Autodesk Inventor part; units mm, degrees
ref_plane "YZ Plane" through (0, 0, 0) normal (1, 0, 0) x (0, 1, 0)
ref_plane "XZ Plane" through (0, 0, 0) normal (0, 1, 0) x (-1, 0, 0)
ref_plane "XY Plane" through (0, 0, 0) normal (0, 0, 1) x (1, 0, 0)
sketch "Sketch1" plane through (0, 0, 0) normal (0, 1, 0) x (-1, 0, 0)
  line L0 (0, 0) -> (25, 0)
  line L1 (0, -25) -> (0, 0)
  line L2 (25, 0) -> (50, 0)
  circle A0 centre (37.5, -12.5) radius 1.5
  circle A1 centre (12.5, -12.5) radius 1.5
  circle A2 centre (12.5, -37.5) radius 1.5
  line L3 (0, 0) -> (0, -25.5)
  line L4 (50, 0) -> (51, 0)
  line L5 (46.5711, -25.5) -> (39.5, -25.5)
  line L6 (25.5, -39.5) -> (25.5, -46.5711)
  line L7 (0, 0) -> (0, -65)
  line L8 (0, 0) -> (65, 0)
  line L9 (65, 0) -> (0, -65)
  line L10 (25.5, 0) -> (25.5, 5)
  line L11 (25.5, 5) -> (33.9376, 5)
  line L12 (0, -25.5) -> (-5, -25.5)
  line L13 (-5, -25.5) -> (-5, -33.9376)
  line L14 (32.5, -32.5) -> (36.0355, -36.0355)
  line L15 (36.0355, -36.0355) -> (25.5, -46.5711)
  line L16 (36.0355, -36.0355) -> (46.5711, -25.5)
  line L17 (28.9376, 0) -> (33.9376, 5)
  line L18 (-5, -33.9376) -> (0, -28.9376)
  line L19 (12.5, -12.5) -> (12.5, -37.5)
  line L20 (12.5, -12.5) -> (37.5, -12.5)
  line L21 (33.9376, 5) -> (38.9376, 0)
  line L22 (25.5, 5) -> (20.5, 0)
  line L23 (-5, -25.5) -> (0, -20.5)
  line L24 (-5, -33.9376) -> (0, -38.9376)
  line L25 (25.5, -46.5711) -> (18.4289, -46.5711)
  line L26 (46.5711, -25.5) -> (46.5711, -18.4289)
  line L27 (46.5711, -18.4289) -> (39.5, -25.5)
  line L28 (25.5, -39.5) -> (18.4289, -46.5711)
  line L29 (0, -20.5) -> (0, -25.5)
  line L30 (25.5, 0) -> (20.5, 0)
  line L31 (0, -28.9376) -> (0, -38.9376)
  line L32 (0, -20.5) -> (0, -25.5)
  line L33 (0, -25.5) -> (0, -28.9376)
  line L34 (0, -28.9376) -> (0, -38.9376)
  line L35 (-5, -33.9376) -> (0, -38.9376)
  line L36 (0, -38.9376) -> (0, -28.9376)
  line L37 (0, -28.9376) -> (-5, -33.9376)
  dimension "d36" = 25
  dimension "d38" = 25
  dimension "d42" = 3
  dimension "d43" = 3
  dimension "d44" = 3
  dimension "d45" = 25.5
  dimension "d47" = 1
  dimension "d51" = 65
  dimension "d52" = 65
  dimension "d54" = 5
  dimension "d55" = 5
  dimension "d56" = 5
extrude "Extrusion5" add sketch "Sketch1" along normal blind 2.5 contours L0 L2 L4 L8 L9 L7 L3 L1 | L22 L10 L2 L0 | L1 L3 L12 L23 | L21 L2 L17 | L18 L7 L24 | L9 L6 L25 | L26 L5 L9
extrude "Extrusion6" add sketch "Sketch1" along normal blind 8 contours L11 L17 L2 L10 | L12 L7 L18 L13 | L9 L14 L15 L6 | L9 L5 L16 L14
properties part number "stencil"
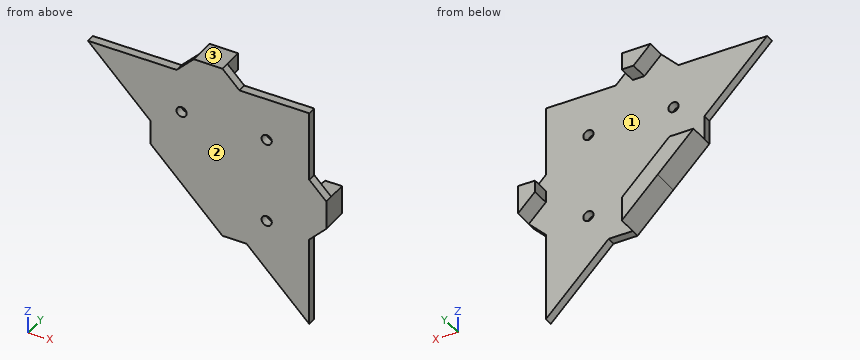
Design review of the part built by this model. Coordinates are the model's own, in mm. Face numbers are marked on the shaded views. Coordinates: 2 decimals unless noted, no trailing zeros. Order: outer loops, then holes, each group sorted by start corner. A loop starts at its lowest first (then second) coordinate and runs counter-clockwise, first axis right, second up. Notation, with made-up numbers: (32, -23.5) -> (52, -23.5) arc R5 cw to (52, -14.5) -> close; hole circle Ø4 at (-1, 80). An arc over 180 degrees is marked (long way). One line per item, written item: value.
1) We need section B-B, the plane z = -12.5. Give the boundary of the cut face in (x, y), then the cut area to 3 significant figures.
Output values:
outline: (-52.5, 0) -> (-39, 0) -> (-39, 2.5) -> (-52.5, 2.5) -> close; (-36, 0) -> (-14, 0) -> (-14, 2.5) -> (-36, 2.5) -> close; (-11, 0) -> (0, 0) -> (0, 2.5) -> (-11, 2.5) -> close
area: 116 mm2
2) Clearance check with flat-ended pins moving along their axes: P1, Ø4, axis at y = 5, z = 3, coming from the +X side; P2, Ø1.2, axis at x = -46.5, y = 2, coming from the +Z side; P3, Ø2.5, axis at x = 3.5, y = 6, coming from the +Z side; P4, Ø1.8, axis at x = -37.5, z = -12.5, coming from the +Y side. State where each tip first meets the part, or that it passes through.
Output values:
P1: stops at x = -25.5
P2: stops at z = 0
P3: stops at z = -25.5
P4: passes through
3) To check wall thickness, follow probe 1 along X at (y, z) = (0.9, -12.5); probe 2 along Y at (x, z) = (-59.5, -3); probe 3 along Z at (x, y) = (-37.5, 1.8). State the ranges of each line that lie inside material, in increasing order. Write a range as [from, to].
Output values:
probe 1: x = [-52.5, -39], [-36, -14], [-11, 0]
probe 2: y = [0, 2.5]
probe 3: z = [-34.57, -14], [-11, 1.44]
4) We need section D-D, the plane x = -12.5. Give the boundary of the cut face in (y, z).
Output values:
outline: (0, -52.5) -> (2.5, -52.5) -> (2.5, -39) -> (0, -39) -> close; (0, -36) -> (2.5, -36) -> (2.5, -14) -> (0, -14) -> close; (0, -11) -> (2.5, -11) -> (2.5, 0) -> (0, 0) -> close
5) Draft analysis for pull direction Z (two halves, no side actions). For the marked faces 1, 2 and 3, state which applies: +Z half, -Z half, draft (parallel to the pull), parting line (faces both ways), or undercut.
Output values:
face 1: undercut
face 2: draft
face 3: +Z half
6) We need section C-C, the plane x = -38. Give the boundary of the cut face in (y, z).
Output values:
outline: (0, -34.07) -> (8, -34.07) -> (8, -27) -> (2.5, -27) -> (2.5, -13.91) -> (0, -13.91) -> close; (0, -11.09) -> (2.5, -11.09) -> (2.5, 0.94) -> (0, 0.94) -> close
7) We need section A-A, the plane y = 4. Give the boundary of the cut face in (x, z).
Output values:
outline: (-46.57, -25.5) -> (-36.04, -36.04) -> (-25.5, -46.57) -> (-25.5, -39.5) -> (-39.5, -25.5) -> close; (-33.94, 5) -> (-28.94, 0) -> (-25.5, 0) -> (-25.5, 5) -> close; (0, -28.94) -> (5, -33.94) -> (5, -25.5) -> (0, -25.5) -> close
